The model under review builds one solid part; all positions refer to its coordinate system, in mm. A direction names the side the tool comes from. Coordinates: 2 decimals unless noted, no trailing zeros. Write each loop counter-clockwise with the first axis right and the second up, starting at its lowest first coordinate (ties: lowest second). Pieces come first, ordered by that corner, then holes.
```python
from build123d import *

# Parameters (mm, degrees)
SKETCH1_W           = 500
SKETCH1_H           = 75
BOSS_EXTRUDE1_DEPTH = 5
SKETCH2_W           = 33.5
SKETCH2_H           = 58.5
SKETCH2_H_2         = 58.503478076
CUT_EXTRUDE1_DEPTH  = 5
SKETCH3_W           = 50
SKETCH3_H           = 75
SKETCH3_W_2         = 33.5
SKETCH3_H_2         = 58.5
SKETCH3_H_3         = 58.503478076
BOSS_EXTRUDE4_DEPTH = 25
SKETCH5_W           = 50
SKETCH5_H           = 75
SKETCH5_W_2         = 33.5
SKETCH5_H_2         = 58.5
SKETCH5_H_3         = 58.503478076
BOSS_EXTRUDE5_DEPTH = 14
FILLET1_R           = 10
FILLET2_R           = 10
SKETCH6_W           = 80
SKETCH6_H           = 60
CUT_EXTRUDE3_DEPTH  = 380
FILLET3_R           = 10


with BuildPart() as part:
    # Sketch1 → Boss-Extrude1 (new body)
    with BuildSketch(Plane.XY):
        Rectangle(SKETCH1_W, SKETCH1_H)
    extrude(amount=BOSS_EXTRUDE1_DEPTH)

    # Sketch2 → Cut-Extrude1 (cut)
    with BuildSketch(Plane.XY.offset(5)):
        with Locations((-99.970770454, 0)):
            Rectangle(SKETCH2_W, SKETCH2_H)
        with Locations((100, 0)):
            Rectangle(SKETCH2_W, SKETCH2_H_2)
    extrude(amount=-CUT_EXTRUDE1_DEPTH, mode=Mode.SUBTRACT)

    # Sketch3 → Boss-Extrude4 (add)
    with BuildSketch(Plane.XY.offset(5)):
        with Locations((-99.970770454, 0)):
            Rectangle(SKETCH3_W, SKETCH3_H)
        with Locations((-99.970770454, 0)):
            Rectangle(SKETCH3_W_2, SKETCH3_H_2, mode=Mode.SUBTRACT)
        with Locations((100, 0)):
            Rectangle(SKETCH3_W, SKETCH3_H)
        with Locations((100, 0)):
            Rectangle(SKETCH3_W_2, SKETCH3_H_3, mode=Mode.SUBTRACT)
    extrude(amount=BOSS_EXTRUDE4_DEPTH)

    # Sketch5 → Boss-Extrude5 (add)
    with BuildSketch(Plane(origin=(0, 0, 0), x_dir=(-1, 0, 0), z_dir=(0, 0, -1))):
        with Locations((99.970770454, 0)):
            Rectangle(SKETCH5_W, SKETCH5_H)
        with Locations((99.970770454, 0)):
            Rectangle(SKETCH5_W_2, SKETCH5_H_2, mode=Mode.SUBTRACT)
        with Locations((-100, 0)):
            Rectangle(SKETCH5_W, SKETCH5_H)
        with Locations((-100, 0)):
            Rectangle(SKETCH5_W_2, SKETCH5_H_3, mode=Mode.SUBTRACT)
    extrude(amount=BOSS_EXTRUDE5_DEPTH)

    # Fillet1
    fillet1_edges = [part.edges().sort_by_distance(p)[0] for p in [
        (75, 0, 0),
        (125, 0, 0),
        (-74.970770454, 0, 5),
        (-124.970770454, 0, 5),
        (125, 0, 5),
        (75, 0, 5),
        (250, -37.5, 2.5),
        (-250, -37.5, 2.5),
        (-250, 37.5, 2.5),
        (250, 37.5, 2.5),
        (-74.970770454, 0, 0),
    ]]
    fillet(fillet1_edges, radius=FILLET1_R)

    # Fillet2
    fillet2_edges = [part.edges().sort_by_distance(p)[0] for p in [
        (-124.970770454, 0, 0),
    ]]
    fillet(fillet2_edges, radius=FILLET2_R)

    # Sketch6 → Cut-Extrude3 (cut)
    with BuildSketch(Plane.XY.offset(5)):
        Rectangle(SKETCH6_W, SKETCH6_H)
    extrude(amount=-CUT_EXTRUDE3_DEPTH, mode=Mode.SUBTRACT)

    # Fillet3
    fillet3_edges = [part.edges().sort_by_distance(p)[0] for p in [
        (40, 30, 2.5),
        (40, -30, 2.5),
        (-40, -30, 2.5),
        (-40, 30, 2.5),
    ]]
    fillet(fillet3_edges, radius=FILLET3_R)


solid = part.part
```
Item 1: To check wall thickness, follow line 1 along X through (y, z) = (-5, 26); line 2 along X through (y, z) = (5, 14); line 3 along Y through (x, z) = (-93, 22). State the ranges of each line that lie inside material, in increasing order.
Solved:
line 1: x = -124.97 to -116.72, -83.22 to -74.97, 75 to 83.25, 116.75 to 125
line 2: x = -125.02 to -116.72, -83.22 to -74.92, 74.95 to 83.25, 116.75 to 125.05
line 3: y = -37.5 to -29.25, 29.25 to 37.5
Item 2: Take a section at C-C, the plane x = 55. Write out the cut boundary in (y, z), plus the area to 3 significant figures.
Solved:
outline: (-37.5, 0) - (37.5, 0) - (37.5, 5) - (-37.5, 5) - close
area: 375 mm2
Item 3: Machinability: for faces 5 (the face through (-83.221, 0, 8)), 6 (the face through (72.15, 0.52, -3.01)), 7 (the face through (75, -1, 22)), 8 (the face through (192, 1, 5)), 9 (the face through (-124.971, -1, 22)), which of the approach directions +Z, -Z, +X, -X, +Y, -Y give a long, thin tool a straight path to every point of the face, cutting with its end or side? Answer none if there is none.
Solved:
face 5: +Z, -Z
face 6: -Z, +Y, -Y
face 7: +Z, +Y, -Y
face 8: +Z, +X, +Y, -Y
face 9: +Z, -X, +Y, -Y
Item 4: Mouldability with a two-part tool opening along X and no side actions: class faces 1 (the face through (100, -29.252, 8)), 2 (the face through (192, 1, 0)), 3 (the face through (-247.15, 34.49, 2.54)), 4 (the face through (36.99, -27.15, 2.46)) as pulls with the +X half, pulls with the -X half, needs draft (parallel to the pull), parting line crosses it, or undercut.
Solved:
face 1: undercut
face 2: needs draft
face 3: pulls with the -X half
face 4: undercut
Item 5: For pin 1 (4.5 mm diameter, centred on y = -18.5, z = -11.5, fed in from +X); pin 2 (12 mm diameter, centred on y = 4.5, z = 24, fed in from -X); pin 3 (4 mm diameter, centred on x = 65.5, y = -4.5, fed in from +Z), all flat-tipped, find the tip position at first contact; note any pin that passes through.
Solved:
pin 1: stops at x = 125.03
pin 2: stops at x = -124.97
pin 3: stops at z = 5.32
Item 6: Take a section at A-A, the plane z = 25. Write out the cut boundary in (x, y).
Solved:
outline: (-124.97, -37.5) - (-74.97, -37.5) - (-74.97, 37.5) - (-124.97, 37.5) - close; (75, -37.5) - (125, -37.5) - (125, 37.5) - (75, 37.5) - close; hole (-116.72, -29.25) - (-83.22, -29.25) - (-83.22, 29.25) - (-116.72, 29.25) - close; hole (83.25, -29.25) - (116.75, -29.25) - (116.75, 29.25) - (83.25, 29.25) - close
Item 7: Take a section at B-B, the plane y = -9. Count the separate pieces of the cut face and the enclosed holes in it, plus the area to 3 significant figures.
Solved:
separate pieces: 4
enclosed holes: 0
area: 3,220 mm2
